Can you work these out from the model? Positions are in its coordinate system, mm. Face numbers are marked on the shaded views. Round coordinates to 2 decimals unless told otherwise and drop trailing zeros. Write each loop counter-clockwise with the first axis right and the second up, starting at its lowest first coordinate (ties: lowest second). Pieces come first, ordered by that corner, then holes. Notation, with made-up numbers: (-32, 87) -> (2, 87) arc R32 ccw to (2, 126) -> close; hole circle Ø11 at (63, 26.25). An arc over 180 degrees is marked (long way). Write item = value, one per line. Start each with the question number.
1) Imagine slicing it at A-A, the plane y = 0.75. Please give me the cut outline in (x, z).
2) Thinking about a two-plate mould opening in Z: for the marked faces 1 and 2, which applies, +Z half, -Z half, draft (parallel to the pull), parting line (faces both ways), or undercut?
3) Imagine slicing it at D-D, the plane x = 30.95. Please give me the cut outline in (y, z).
4) If I drill on line 1 (X direction, y = 1.95, z = -52.09); line 2 (X direction, y = 1.15, z = -26.5); line 3 (Z direction, x = 13, y = 4.5), over which ranges is the centre line in solid material (lowest first)?
5) I'm going to push flat-ended pins straight in: pin 1 (0.5 mm diameter, centred on y = 4.5, z = -53.5, fed in from -X); pin 2 (0.8 mm diameter, centred on x = 33.5, y = 3.5, fed in from +Z); pin 3 (1 mm diameter, centred on x = 5, z = -45, fed in from +Y). Where does each tip first touch, or does it pass through?
6) Imagine slicing it at B-B, the plane x = 11.5. Please give me the cut outline in (y, z).
7) Imagine slicing it at C-C, the plane z = -44. Please give me the cut outline in (x, y), then the cut area to 3 significant figures.
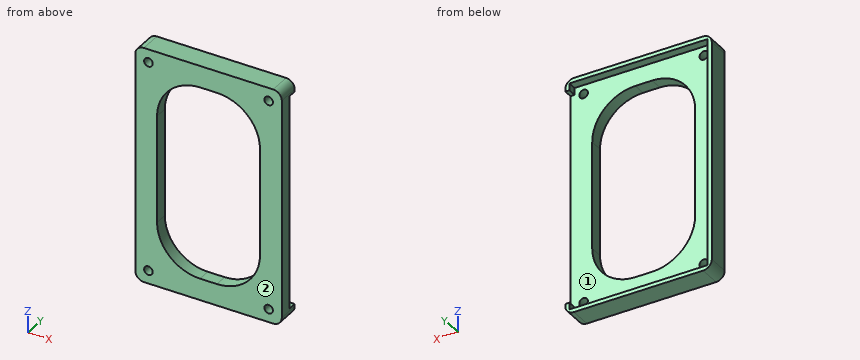
from build123d import *

# Parameters (mm, degrees)
SKETCH_1_W          = 34
SKETCH_1_H          = 55.14
EXTRUDE_1_DEPTH     = 5
SKETCH_2_W          = 32.1
SKETCH_2_H          = 53.24
CUT_EXTRUDE_1_DEPTH = 2
SKETCH_3_W          = 50
SKETCH_3_H          = 10
CUT_EXTRUDE_2_DEPTH = 2
FILLET_3_R          = 2
FILLET_4_R          = 2
FILLET_5_R          = 2
FILLET_6_R          = 2
SKETCH_5_R          = 1
CUT_EXTRUDE_3_DEPTH = 5
CUT_EXTRUDE_5_DEPTH = 5
SKETCH_7_W          = 24.577640881
SKETCH_7_H          = 46.089683544
EXTRUDE_3_DEPTH     = 3
SKETCH_8_W          = 20
SKETCH_8_H          = 6
EXTRUDE_5_DEPTH     = 5
SKETCH_9_W          = 20
SKETCH_9_H          = 6
EXTRUDE_6_DEPTH     = 5
CUT_EXTRUDE_6_DEPTH = 65.972452624
FILLET_7_R          = 2
FILLET_8_R          = 2
FILLET_9_R          = 2
FILLET_10_R         = 2
FILLET_11_R         = 2
FILLET_12_R         = 2
FILLET_13_R         = 2
FILLET_14_R         = 2
SKETCH_11_W         = 2
SKETCH_11_H         = 50
EXTRUDE_7_DEPTH     = 3
SKETCH_12_W         = 87.292454737
SKETCH_12_H         = 120.507181867
CUT_EXTRUDE_7_DEPTH = 10
SKETCH_13_W         = 23.9
SKETCH_13_H         = 45.04
CUT_EXTRUDE_8_DEPTH = 10
FILLET_15_R         = 10
FILLET_16_R         = 10
FILLET_17_R         = 10
FILLET_18_R         = 10


with BuildPart() as part:
    # 草图1 → 凸台-拉伸1 (new body)
    with BuildSketch(Plane(origin=(0, 0, 0), x_dir=(1, 0, 0), z_dir=(0, 1, 0))):
        with Locations((17, 27.57)):
            Rectangle(SKETCH_1_W, SKETCH_1_H)
    extrude(amount=EXTRUDE_1_DEPTH)

    # 草图2 → 切除-拉伸1 (cut)
    with BuildSketch(Plane(origin=(0, 5, 0), x_dir=(1, 0, 0), z_dir=(0, 1, 0))):
        with Locations((17, 27.57)):
            Rectangle(SKETCH_2_W, SKETCH_2_H)
    extrude(amount=-CUT_EXTRUDE_1_DEPTH, mode=Mode.SUBTRACT)

    # 草图3 → 切除-拉伸2 (cut)
    with BuildSketch(Plane(origin=(34, 0, 0), x_dir=(0, 0, -1), z_dir=(1, 0, 0))):
        with Locations((27.57, 5)):
            Rectangle(SKETCH_3_W, SKETCH_3_H)
    extrude(amount=-CUT_EXTRUDE_2_DEPTH, mode=Mode.SUBTRACT)

    # 圆角3
    fillet_3_edges = [part.edges().sort_by_distance(p)[0] for p in [
        (0, 2.5, 0),
    ]]
    fillet(fillet_3_edges, radius=FILLET_3_R)

    # 圆角4
    fillet_4_edges = [part.edges().sort_by_distance(p)[0] for p in [
        (0, 2.5, -55.14),
    ]]
    fillet(fillet_4_edges, radius=FILLET_4_R)

    # 圆角5
    fillet_5_edges = [part.edges().sort_by_distance(p)[0] for p in [
        (34, 2.5, -55.14),
    ]]
    fillet(fillet_5_edges, radius=FILLET_5_R)

    # 圆角6
    fillet_6_edges = [part.edges().sort_by_distance(p)[0] for p in [
        (34, 2.5, 0),
    ]]
    fillet(fillet_6_edges, radius=FILLET_6_R)

    # 草图5 → 切除-拉伸3 (cut)
    with BuildSketch(Plane(origin=(0, 3, 0), x_dir=(1, 0, 0), z_dir=(0, 1, 0))):
        with Locations(Location((3.05, 52.09, 0), (0, 0, 270))):
            Circle(SKETCH_5_R)
        with Locations(Location((3.05, 3.05, 0), (0, 0, 90))):
            Circle(SKETCH_5_R)
        with Locations(Location((30.95, 3.05, 0), (0, 0, 270))):
            Circle(SKETCH_5_R)
        with Locations(Location((30.95, 52.09, 0), (0, 0, 90))):
            Circle(SKETCH_5_R)
    extrude(amount=-CUT_EXTRUDE_3_DEPTH, mode=Mode.SUBTRACT)

    # 草图6 → 切除-拉伸5 (cut)
    with BuildSketch(Plane(origin=(0, 3, 0), x_dir=(1, 0, 0), z_dir=(0, 1, 0))):
        with BuildLine():
            ThreePointArc((5.05, 49.09), (5.342893219, 49.797106781), (6.05, 50.09))
            Line((6.05, 50.09), (6.254717451, 50.09))
            ThreePointArc((6.254717451, 50.09), (6.961824232, 49.797106781), (7.254717451, 49.09))
            Line((7.254717451, 49.09), (7.254717451, 6.05))
            ThreePointArc((7.254717451, 6.05), (6.961824232, 5.342893219), (6.254717451, 5.05))
            Line((6.254717451, 5.05), (6.05, 5.05))
            ThreePointArc((6.05, 5.05), (5.342893219, 5.342893219), (5.05, 6.05))
            Line((5.05, 6.05), (5.05, 49.09))
        make_face()
        with BuildLine():
            ThreePointArc((10.05, 49.09), (10.342893219, 49.797106781), (11.05, 50.09))
            Line((11.05, 50.09), (11.254717451, 50.09))
            ThreePointArc((11.254717451, 50.09), (11.961824232, 49.797106781), (12.254717451, 49.09))
            Line((12.254717451, 49.09), (12.254717451, 6.05))
            ThreePointArc((12.254717451, 6.05), (11.961824232, 5.342893219), (11.254717451, 5.05))
            Line((11.254717451, 5.05), (11.05, 5.05))
            ThreePointArc((11.05, 5.05), (10.342893219, 5.342893219), (10.05, 6.05))
            Line((10.05, 6.05), (10.05, 49.09))
        make_face()
        with BuildLine():
            ThreePointArc((20.05, 49.09), (20.342893219, 49.797106781), (21.05, 50.09))
            Line((21.05, 50.09), (21.254717451, 50.09))
            ThreePointArc((21.254717451, 50.09), (21.961824232, 49.797106781), (22.254717451, 49.09))
            Line((22.254717451, 49.09), (22.254717451, 6.05))
            ThreePointArc((22.254717451, 6.05), (21.961824232, 5.342893219), (21.254717451, 5.05))
            Line((21.254717451, 5.05), (21.05, 5.05))
            ThreePointArc((21.05, 5.05), (20.342893219, 5.342893219), (20.05, 6.05))
            Line((20.05, 6.05), (20.05, 49.09))
        make_face()
        with BuildLine():
            ThreePointArc((26.05, 5.05), (25.342893219, 5.342893219), (25.05, 6.05))
            Line((25.05, 6.05), (25.05, 49.09))
            ThreePointArc((25.05, 49.09), (25.342893219, 49.797106781), (26.05, 50.09))
            Line((26.05, 50.09), (26.254717451, 50.09))
            ThreePointArc((26.254717451, 50.09), (26.961824232, 49.797106781), (27.254717451, 49.09))
            Line((27.254717451, 49.09), (27.254717451, 6.05))
            ThreePointArc((27.254717451, 6.05), (26.961824232, 5.342893219), (26.254717451, 5.05))
            Line((26.254717451, 5.05), (26.05, 5.05))
        make_face()
        with BuildLine():
            Line((15.05, 49.09), (15.05, 6.05))
            ThreePointArc((15.05, 6.05), (15.342893219, 5.342893219), (16.05, 5.05))
            Line((16.05, 5.05), (16.254717451, 5.05))
            ThreePointArc((16.254717451, 5.05), (16.961824232, 5.342893219), (17.254717451, 6.05))
            Line((17.254717451, 6.05), (17.254717451, 49.09))
            ThreePointArc((17.254717451, 49.09), (16.961824232, 49.797106781), (16.254717451, 50.09))
            Line((16.254717451, 50.09), (16.05, 50.09))
            ThreePointArc((16.05, 50.09), (15.342893219, 49.797106781), (15.05, 49.09))
        make_face()
    extrude(amount=-CUT_EXTRUDE_5_DEPTH, mode=Mode.SUBTRACT)

    # 草图7 → 凸台-拉伸3 (add)
    with BuildSketch(Plane.XZ):
        with Locations((15.625766317, -27.57)):
            Rectangle(SKETCH_7_W, SKETCH_7_H)
    extrude(amount=-EXTRUDE_3_DEPTH)

    # 草图8 → 凸台-拉伸5 (add)
    with BuildSketch(Plane.XZ):
        with Locations((17, -3)):
            Rectangle(SKETCH_8_W, SKETCH_8_H)
    extrude(amount=EXTRUDE_5_DEPTH)

    # 草图9 → 凸台-拉伸6 (add)
    with BuildSketch(Plane.XZ):
        with Locations((17, -52.14)):
            Rectangle(SKETCH_9_W, SKETCH_9_H)
    extrude(amount=EXTRUDE_6_DEPTH)

    # 草图10 → 切除-拉伸6 (cut, through all)
    with BuildSketch(Plane(origin=(0, 0, -55.14), x_dir=(-1, 0, 0), z_dir=(0, 0, -1))):
        with BuildLine():
            ThreePointArc((-8, -2.5), (-11.414213562, -1.085786438), (-10, -4.5))
            Line((-10, -4.5), (-10, -2.5))
            Line((-10, -2.5), (-8, -2.5))
        make_face()
        with BuildLine():
            Line((-10, -2.5), (-10, -4.5))
            ThreePointArc((-10, -4.5), (-8.585786438, -3.914213562), (-8, -2.5))
            Line((-8, -2.5), (-10, -2.5))
        make_face()
        with BuildLine():
            ThreePointArc((-26, -2.5), (-25.414213562, -3.914213562), (-24, -4.5))
            Line((-24, -4.5), (-24, -2.5))
            Line((-24, -2.5), (-26, -2.5))
        make_face()
        with BuildLine():
            Line((-24, -2.5), (-24, -4.5))
            ThreePointArc((-24, -4.5), (-22.585786438, -3.914213562), (-22, -2.5))
            ThreePointArc((-22, -2.5), (-24, -0.5), (-26, -2.5))
            Line((-26, -2.5), (-24, -2.5))
        make_face()
    extrude(amount=-CUT_EXTRUDE_6_DEPTH, mode=Mode.SUBTRACT)

    # 圆角7
    fillet_7_edges = [part.edges().sort_by_distance(p)[0] for p in [
        (7, -5, -52.14),
    ]]
    fillet(fillet_7_edges, radius=FILLET_7_R)

    # 圆角8
    fillet_8_edges = [part.edges().sort_by_distance(p)[0] for p in [
        (7, 0, -52.14),
    ]]
    fillet(fillet_8_edges, radius=FILLET_8_R)

    # 圆角9
    fillet_9_edges = [part.edges().sort_by_distance(p)[0] for p in [
        (27, -5, -52.14),
    ]]
    fillet(fillet_9_edges, radius=FILLET_9_R)

    # 圆角10
    fillet_10_edges = [part.edges().sort_by_distance(p)[0] for p in [
        (27, 0, -52.14),
    ]]
    fillet(fillet_10_edges, radius=FILLET_10_R)

    # 圆角11
    fillet_11_edges = [part.edges().sort_by_distance(p)[0] for p in [
        (7, -5, -3),
    ]]
    fillet(fillet_11_edges, radius=FILLET_11_R)

    # 圆角12
    fillet_12_edges = [part.edges().sort_by_distance(p)[0] for p in [
        (7, 0, -3),
    ]]
    fillet(fillet_12_edges, radius=FILLET_12_R)

    # 圆角13
    fillet_13_edges = [part.edges().sort_by_distance(p)[0] for p in [
        (27, -5, -3),
    ]]
    fillet(fillet_13_edges, radius=FILLET_13_R)

    # 圆角14
    fillet_14_edges = [part.edges().sort_by_distance(p)[0] for p in [
        (27, 0, -3),
    ]]
    fillet(fillet_14_edges, radius=FILLET_14_R)

    # 草图11 → 凸台-拉伸7 (add)
    with BuildSketch(Plane.XZ):
        with Locations((33, -27.57)):
            Rectangle(SKETCH_11_W, SKETCH_11_H)
    extrude(amount=-EXTRUDE_7_DEPTH)

    # 草图12 → 切除-拉伸7 (cut)
    with BuildSketch(Plane.XZ):
        with Locations((-3.68135744, 1.129600161)):
            Rectangle(SKETCH_12_W, SKETCH_12_H)
    extrude(amount=CUT_EXTRUDE_7_DEPTH, mode=Mode.SUBTRACT)

    # 草图13 → 切除-拉伸8 (cut)
    with BuildSketch(Plane.XZ):
        with Locations((17, -27.57)):
            Rectangle(SKETCH_13_W, SKETCH_13_H)
    extrude(amount=-CUT_EXTRUDE_8_DEPTH, mode=Mode.SUBTRACT)

    # 圆角15
    fillet_15_edges = [part.edges().sort_by_distance(p)[0] for p in [
        (28.95, 1.5, -50.09),
    ]]
    fillet(fillet_15_edges, radius=FILLET_15_R)

    # 圆角16
    fillet_16_edges = [part.edges().sort_by_distance(p)[0] for p in [
        (5.05, 1.5, -50.09),
    ]]
    fillet(fillet_16_edges, radius=FILLET_16_R)

    # 圆角17
    fillet_17_edges = [part.edges().sort_by_distance(p)[0] for p in [
        (28.95, 1.5, -5.05),
    ]]
    fillet(fillet_17_edges, radius=FILLET_17_R)

    # 圆角18
    fillet_18_edges = [part.edges().sort_by_distance(p)[0] for p in [
        (5.05, 1.5, -5.05),
    ]]
    fillet(fillet_18_edges, radius=FILLET_18_R)


solid = part.part
Reported:
q1.outline = (0, -53.14) arc R2 ccw to (2, -55.14) -> (32, -55.14) arc R2 ccw to (34, -53.14) -> (34, -2) arc R2 ccw to (32, 0) -> (2, 0) arc R2 ccw to (0, -2) -> close; hole circle Ø2 at (3.05, -52.09); hole circle Ø2 at (3.05, -3.05); hole (5.05, -40.09) arc R10 ccw to (15.05, -50.09) -> (18.95, -50.09) arc R10 ccw to (28.95, -40.09) -> (28.95, -15.05) arc R10 ccw to (18.95, -5.05) -> (15.05, -5.05) arc R10 ccw to (5.05, -15.05) -> close; hole circle Ø2 at (30.95, -52.09); hole circle Ø2 at (30.95, -3.05)
q2.face_1 = undercut
q2.face_2 = draft
q3.outline = (0, -55.14) -> (5, -55.14) -> (5, -54.19) -> (3, -54.19) -> (3, -53.09) -> (0, -53.09) -> close; (0, -51.09) -> (3, -51.09) -> (3, -4.05) -> (0, -4.05) -> close; (0, -2.05) -> (3, -2.05) -> (3, -0.95) -> (5, -0.95) -> (5, 0) -> (0, 0) -> close
q4.line_1 = 0 to 2.05, 4.05 to 29.95, 31.95 to 34
q4.line_2 = 0 to 5.05, 28.95 to 34
q4.line_3 = -55.14 to -54.19, -0.95 to 0
q5.pin_1 = 0
q5.pin_2 = -0.33
q5.pin_3 = 3
q6.outline = (0, -55.14) -> (5, -55.14) -> (5, -54.19) -> (3, -54.19) -> (3, -49.44) -> (0, -49.44) -> close; (0, -5.7) -> (3, -5.7) -> (3, -0.95) -> (5, -0.95) -> (5, 0) -> (0, 0) -> close
q7.outline = (0, 0) -> (5.85, 0) -> (5.85, 3) -> (0.95, 3) -> (0.95, 5) -> (0, 5) -> close; (28.15, 0) -> (34, 0) -> (34, 3) -> (28.15, 3) -> close
q7.area = 37.0 mm²
